Geometry check sheet. Reference: the model listing, model coordinates, mm. A direction names the side the tool comes from. Round coordinates to 2 decimals unless told otherwise and drop trailing zeros. Loops run counter-clockwise (first coordinate to the right, second up) from the corner with the lowest first, then second, coordinate; pieces in that order, holes last. Notation, with made-up numbers: (-26.75, -6.75) -> (10.25, -6.75) arc R19 ccw to (10.25, 17.25) -> close; hole circle Ø2 at (24.25, -25). An arc over 180 degrees is marked (long way). Use a Markdown table: item, result. Add a question column.
Q1. Sectioned sample at C-C, the plane x = 0. Enter the section's corners in (y, z), then the cut area to 3 significant figures.
Q2. Sectioned sample at A-A, the plane z = 7.5. Enter the section's corners in (x, y) (3 decimals), then the cut area to 3 significant figures.
Q3. Sectioned sample at D-D, the plane y = 5.5. Enter the section's corners in (x, z), then the cut area to 3 significant figures.
Q4. Gauge pin test, flat ends, axial feed: P1, Ø1.5, axis at y = 4, z = 3.5, coming from the -X side; P2, Ø4, axis at x = -9.5, z = 10.5, coming from the +Y side; P3, Ø2, axis at y = 3, z = 1.5, coming from the +X side; P4, Ø2.5, axis at x = -10.39, z = 7.5, coming from the -Y side. Record the tip position at first contact, or that the pin passes through.
Q5. Set-up check for faces 5 (the face through (-0.1, 4.45, 7.4)), 6 (the face through (-10.3, 1.5, 5.7)), 7 (the face through (10.4, 1.5, 5.7)): record each of +Z, -Z, +X, -X, +Y, -Y from which the full face is reachable in a straight line by a thin tool's end or side.
Q6. Release check for a two-part mould opening along Z. For faces 1 (the face through (0.12, 6.45, 7.4)), 2 (the face through (0, 5, 15)), 3 (the face through (0, 5, 0)), 4 (the face through (11.541, 0.727, 8.382)) record: released by +Z, released by -Z, zero draft, split by the parting line, or undercut.
Q7. Material ranges on L1, parallel to X at y = 0.4, z = 7.5; L2, parallel to X at y = 0.55, z = 7.5; L3, parallel to Y at x = -12.5, z = 6, recorded low to high.
```python
from build123d import *

# Parameters (mm, degrees)
BOSS_EXTRUDE1_DEPTH              = 15
M2_5_CLEARANCE_HOLE1_D           = 2.9
M2_5_CLEARANCE_HOLE1_CSINK_D     = 2.95
M2_5_CLEARANCE_HOLE1_CSINK_ANGLE = 90


with BuildPart() as part:
    # Sketch1 → Boss-Extrude1 (new body)
    with BuildSketch(Plane.XY):
        with BuildLine():
            Line((-14.390422521, 0), (-4.597553697, 0))
            ThreePointArc((-4.597553697, 0), (0, 4.45), (4.597553697, 0))
            Line((4.597553697, 0), (14.390422521, 0))
            Line((14.390422521, 0), (14.390422521, 1.5))
            Line((14.390422521, 1.5), (6.390422521, 1.5))
            ThreePointArc((6.390422521, 1.5), (0, 6.45), (-6.390422521, 1.5))
            Line((-6.390422521, 1.5), (-14.390422521, 1.5))
            Line((-14.390422521, 1.5), (-14.390422521, 0))
        make_face()
    extrude(amount=BOSS_EXTRUDE1_DEPTH)

    # M2.5 Clearance Hole1 (through all)
    with Locations(Plane(origin=(0, 1.5, 0), x_dir=(1, 0, 0), z_dir=(0, 1, 0))):
        with Locations((-10.390422521, -7.5), (10.390422521, -7.5)):
            CounterSinkHole(M2_5_CLEARANCE_HOLE1_D / 2, M2_5_CLEARANCE_HOLE1_CSINK_D / 2, counter_sink_angle=M2_5_CLEARANCE_HOLE1_CSINK_ANGLE)


solid = part.part
```
Values:
| question | item | result |
|---|---|---|
| 1 | outline | (4.45, 0) -> (6.45, 0) -> (6.45, 15) -> (4.45, 15) -> close |
| 1 | area | 30.0 mm^2 |
| 2 | outline | (-14.39, 0) -> (-11.84, 0) -> (-11.84, 1.475) -> (-11.865, 1.5) -> (-14.39, 1.5) -> close; (-8.94, 0) -> (-4.598, 0) arc R4.6 cw to (4.598, 0) -> (8.94, 0) -> (8.94, 1.475) -> (8.915, 1.5) -> (6.39, 1.5) arc R6.6 ccw to (-6.39, 1.5) -> (-8.915, 1.5) -> (-8.94, 1.475) -> close; (11.84, 0) -> (14.39, 0) -> (14.39, 1.5) -> (11.865, 1.5) -> (11.84, 1.475) -> close |
| 2 | area | 49.5 mm^2 |
| 3 | outline | (-3.41, 0) -> (3.41, 0) -> (3.41, 15) -> (-3.41, 15) -> close |
| 3 | area | 102 mm^2 |
| 4 | P1 | x = -5.66 |
| 4 | P2 | y = 1.5 |
| 4 | P3 | x = 6.24 |
| 4 | P4 | through |
| 5 | face 5 | +Z, -Z, -Y |
| 5 | face 6 | +Z, -Z, -X, +Y |
| 5 | face 7 | +Z, -Z, +X, +Y |
| 6 | face 1 | zero draft |
| 6 | face 2 | released by +Z |
| 6 | face 3 | released by -Z |
| 6 | face 4 | undercut |
| 7 | L1 | -14.39 to -11.84, -8.94 to -4.57, 4.57 to 8.94, 11.84 to 14.39 |
| 7 | L2 | -14.39 to -11.84, -8.94 to -4.55, 4.55 to 8.94, 11.84 to 14.39 |
| 7 | L3 | 0 to 1.5 |
